Check sheet for the drawn part. Datum: minimum x, y, z corner. Units: mm. Give positions to 0.01 mm unless a question says otherwise; leave off trailing zeros. Order: outer loops, then holes, each group sorted by start corner. A loop starts at its lowest first (then second) coordinate and runs counter-clockwise, first axis right, second up. Notation, with made-up numbers: (2, 37) - (57, 37) arc R31 ccw to (57, 72) - close; hole circle Ø2 at (-0.75, -30). An arc over 180 degrees is marked (long way). Answer as a JSON object with one key per item and string values. Group by question number.
(1) Thickness scan on line 1 (X direction, y = 42, z = 1.5) (1 decimal); line 2 (X direction, y = 34.5, z = 6.5) (1 decimal); line 3 (Y direction, x = 71, z = 2.5). Record the ranges inside material, lowest first.
(2) Mould release check, pull along Y, two halves, no side actions. Record for the marked faces 1, 2, 3 and 4: +Y half, -Y half, draft (parallel to the pull), parting line (faces both ways), or undercut.
(3) Section check A-A (z = 6.75). Record the boundary of the cut face in (x, y).
(4) Section check B-B (y = 91.5). Record the boundary of the cut face in (x, z), then the cut area to 3 significant figures.
(5) Section check C-C (x = 13). Record the boundary of the cut face in (y, z).
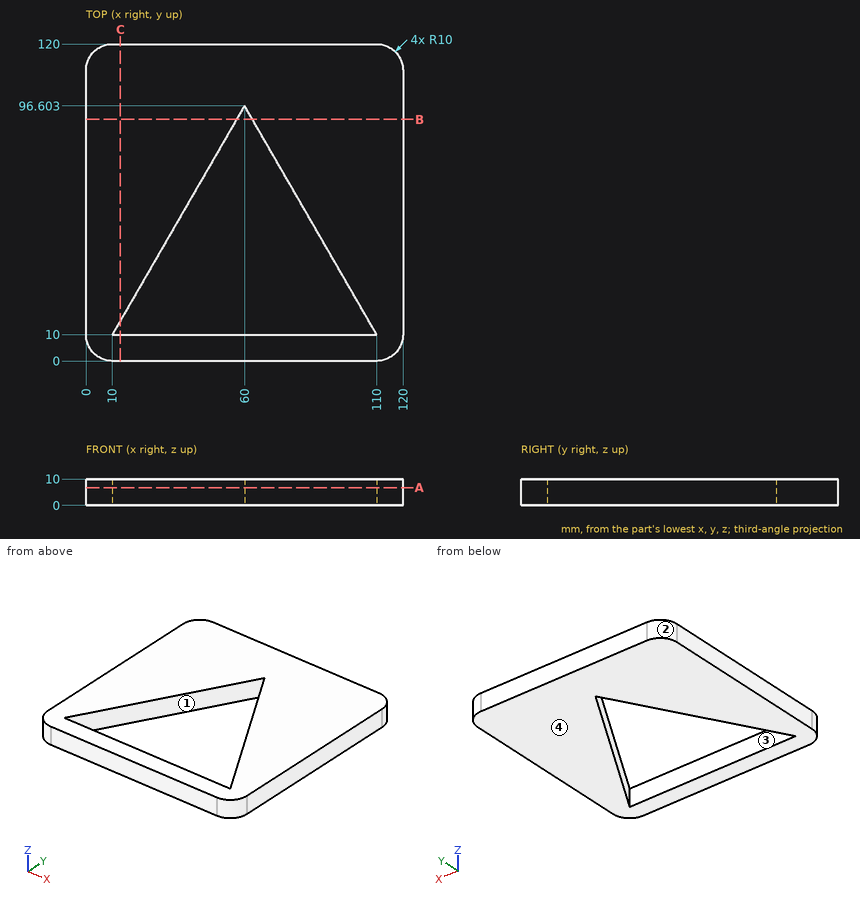
Solutions:
{
 "1": {"line 1": "x = 0 to 28.5, 91.5 to 120", "line 2": "x = 0 to 24.1, 95.9 to 120", "line 3": "y = 0 to 10, 77.55 to 120"},
 "2": {"face 1": "undercut", "face 2": "+Y half", "face 3": "undercut", "face 4": "draft"},
 "3": {"outline": "(0, 10) arc R10 ccw to (10, 0) - (110, 0) arc R10 ccw to (120, 10) - (120, 110) arc R10 ccw to (110, 120) - (10, 120) arc R10 ccw to (0, 110) - close; hole (10, 10) - (110, 10) - (60, 96.6) - close"},
 "4": {"outline": "(0, 0) - (57.05, 0) - (57.05, 10) - (0, 10) - close; (62.95, 0) - (120, 0) - (120, 10) - (62.95, 10) - close", "area": "1,140 mm2"},
 "5": {"outline": "(0, 0) - (10, 0) - (10, 10) - (0, 10) - close; (15.2, 0) - (120, 0) - (120, 10) - (15.2, 10) - close"}
}
